```python
from build123d import *

# Parameters (mm, degrees)
SKETCH2_R           = 2.4
BOSS_EXTRUDE1_DEPTH = 1
SKETCH3_R           = 60
CUT_EXTRUDE1_DEPTH  = 1


with BuildPart() as part:
    # Sketch2 → Boss-Extrude1 (new body)
    with BuildSketch(Plane(origin=(0, 0, 0), x_dir=(1, 0, 0), z_dir=(0, 1, 0))):
        with BuildLine():
            Line((77.497806421, 77.5), (-77.497806421, 77.5))
            ThreePointArc((-77.497806421, 77.5), (-77.498903218, 77.498903218), (-77.5, 77.497806421))
            Line((-77.5, 77.497806421), (-77.5, -77.497806421))
            ThreePointArc((-77.5, -77.497806421), (-77.498903218, -77.498903218), (-77.497806421, -77.5))
            Line((-77.497806421, -77.5), (77.497806421, -77.5))
            ThreePointArc((77.497806421, -77.5), (77.498903218, -77.498903218), (77.5, -77.497806421))
            Line((77.5, -77.497806421), (77.5, 77.497806421))
            ThreePointArc((77.5, 77.497806421), (77.498903218, 77.498903218), (77.497806421, 77.5))
        make_face()
        with Locations(Location((-60.1, -60.1, 0), (0, 0, 270))):
            Circle(SKETCH2_R, mode=Mode.SUBTRACT)
        with Locations(Location((60.1, -60.1, 0), (0, 0, 270))):
            Circle(SKETCH2_R, mode=Mode.SUBTRACT)
        with Locations(Location((-60.1, 60.1, 0), (0, 0, 270))):
            Circle(SKETCH2_R, mode=Mode.SUBTRACT)
        with Locations(Location((60.1, 60.1, 0), (0, 0, 270))):
            Circle(SKETCH2_R, mode=Mode.SUBTRACT)
    extrude(amount=BOSS_EXTRUDE1_DEPTH)

    # Sketch3 → Cut-Extrude1 (cut)
    with BuildSketch(Plane(origin=(0, 1, 0), x_dir=(1, 0, 0), z_dir=(0, 1, 0))):
        with Locations(Location((0, 0, 0), (0, 0, 270))):
            Circle(SKETCH3_R)
    extrude(amount=-CUT_EXTRUDE1_DEPTH, mode=Mode.SUBTRACT)


solid = part.part
```
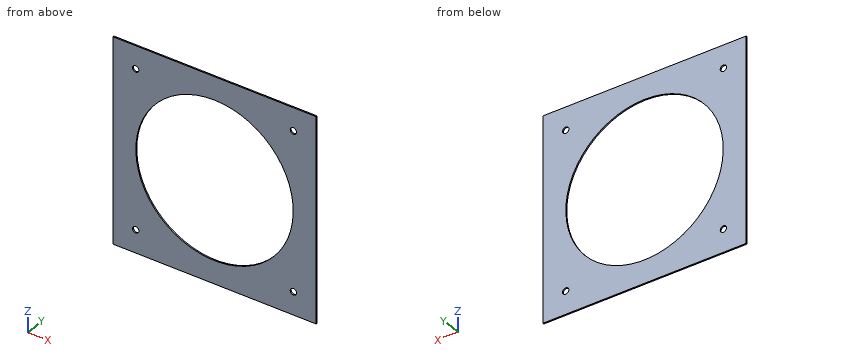
Can you work these out from the model? Positions are in its coordinate system, mm. Round coordinates to 2 decimals unless told otherwise and drop trailing zeros. Loops run counter-clockwise (first coordinate to the right, second up) from the corner with the lowest first, then second, coordinate; pieces in that order, holes last. Notation, with made-up numbers: (54, 56.25) -> (60, 56.25) arc R35 ccw to (60, 93.25) -> close; hole circle Ø7 at (-17.5, 19). An arc over 180 degrees is marked (long way). Answer in a Markdown table with one row per item.
Item 1: Suppose I cut it at B-B, the plane y = 0.65. Give the number of separate pieces and of enclosed holes in the cut face, plus the area to 3 significant figures.
Answer block:
| item | result |
|---|---|
| separate pieces | 1 |
| enclosed holes | 5 |
| area | 12,600 mm² |
Item 2: Suppose I cut it at A-A, the plane z = 0. List the corners of the cut face in (x, y) for me.
Answer block:
| item | result |
|---|---|
| outline | (-77.5, 0) -> (-60, 0) -> (-60, 1) -> (-77.5, 1) -> close; (60, 0) -> (77.5, 0) -> (77.5, 1) -> (60, 1) -> close |
Item 3: If I drill on probe 1 along X at (y, z) = (0.35, 60.1); probe 2 along X at (y, z) = (0.4, 0); probe 3 along Z at (x, y) = (31.5, 0.35), over which ranges is the centre line in solid material (lowest first)?
Answer block:
| item | result |
|---|---|
| probe 1 | -77.5 to -62.5, -57.7 to 57.7, 62.5 to 77.5 |
| probe 2 | -77.5 to -60, 60 to 77.5 |
| probe 3 | -77.5 to -51.07, 51.07 to 77.5 |
Item 4: Suppose I cut it at C-C, the plane x = 6. List the corners of the cut face in (y, z) for me.
Answer block:
| item | result |
|---|---|
| outline | (0, -77.5) -> (1, -77.5) -> (1, -59.7) -> (0, -59.7) -> close; (0, 59.7) -> (1, 59.7) -> (1, 77.5) -> (0, 77.5) -> close |
